Build history of the part. All positions in model axes, mm. Face numbers are marked on the shaded views. A direction names the side the tool comes from. Coordinates: 2 decimals unless noted, no trailing zeros. Loops run counter-clockwise (first coordinate to the right, second up) from the corner with the lowest first, then second, coordinate; pieces in that order, holes last.
Item 1: Drill centre lines: line 1 along Y through (x, z) = (-10.5, 21.5) (3 decimals); line 2 along Y through (x, z) = (35, 21) (3 decimals); line 3 along Y through (x, z) = (-15, 34.5) (3 decimals). Where is each one in solid material? Low to high.
Item 2: Cut at B-B (x = -7.5). List the corners of the cut face in (y, z) (3 decimals), and give its area (3 significant figures).
Item 3: 3-axis set-ups, long thin cutter, end or side, ignore diameter. For the marked faces 1 and 2: which of +Z, -Z, +X, -X, +Y, -Y reach the whole face in a straight line?
Item 4: Flat gauge pins, fed straight in: pin 1 (0.6 mm diameter, centred on x = 35.5, y = 30.5, fed in from +Z); pin 2 (4 mm diameter, centred on x = 41.275, y = -41.275, fed in from +Z). Where does each tip first touch, or does it go through?
Item 5: Cut at A-A (z = 8). Count the separate pieces of the cut face and the enclosed holes in it, and give its area (3 significant figures).
Item 6: Cut at C-C (y = 9). List the corners of the cut face in (x, z) (3 decimals), and give its area (3 significant figures).
Item 7: Mould opens along Y. For the marked faces 3, 4, 5 and 6 say: released by +Y, released by -Y, zero draft, split by the parting line, or undercut.
Item 8: Cut at D-D (z = 33). List the corners of the cut face in (x, y) (1 decimal).
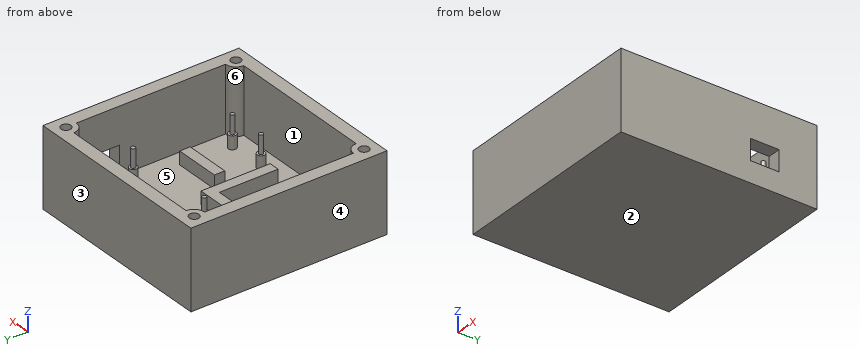
from build123d import *

# Parameters (mm, degrees)
SKETCH1_W           = 95.25
SKETCH1_H           = 95.25
BOSS_EXTRUDE1_DEPTH = 38.1
SHELL1_T            = -6.35
BOSS_EXTRUDE2_DEPTH = 31.75
SKETCH3_R           = 1.905
SKETCH3_R_2         = 1.016
BOSS_EXTRUDE3_DEPTH = 6.35
SKETCH4_R           = 1.016
BOSS_EXTRUDE4_DEPTH = 8.89
SKETCH5_R           = 1.905
SKETCH5_W           = 22.2885
SKETCH5_H           = 5.08
BOSS_EXTRUDE5_DEPTH = 6.35
SKETCH7_R           = 1.016
BOSS_EXTRUDE6_DEPTH = 8.89
SKETCH8_R           = 2.38125
CUT_EXTRUDE1_DEPTH  = 8.89
BOSS_EXTRUDE7_DEPTH = 6.35
SKETCH12_W          = 10.16
SKETCH12_H          = 13.97
CUT_EXTRUDE2_DEPTH  = 6.35


with BuildPart() as part:
    # Sketch1 → Boss-Extrude1 (new body)
    with BuildSketch(Plane.XY):
        Rectangle(SKETCH1_W, SKETCH1_H)
    extrude(amount=BOSS_EXTRUDE1_DEPTH)

    # Shell1
    shell1_openings = [part.faces().sort_by_distance(p)[0] for p in [
        (0, 0, 38.1),
    ]]
    offset(amount=SHELL1_T, openings=shell1_openings, kind=Kind.INTERSECTION)

    # Sketch2 → Boss-Extrude2 (add)
    with BuildSketch(Plane.XY.offset(38.1)):
        with BuildLine():
            Line((-41.275, 41.275), (-36.195, 41.275))
            ThreePointArc((-36.195, 41.275), (-37.682897552, 37.682897552), (-41.275, 36.195))
            Line((-41.275, 36.195), (-41.275, 41.275))
        make_face()
        with BuildLine():
            Line((36.195, 41.275), (41.275, 41.275))
            Line((41.275, 41.275), (41.275, 36.195))
            ThreePointArc((41.275, 36.195), (37.682897552, 37.682897552), (36.195, 41.275))
        make_face()
        with BuildLine():
            Line((41.275, -36.195), (41.275, -41.275))
            Line((41.275, -41.275), (36.195, -41.275))
            ThreePointArc((36.195, -41.275), (37.682897552, -37.682897552), (41.275, -36.195))
        make_face()
        with BuildLine():
            Line((-41.275, -36.195), (-41.275, -41.275))
            Line((-41.275, -41.275), (-36.195, -41.275))
            ThreePointArc((-36.195, -41.275), (-37.682897552, -37.682897552), (-41.275, -36.195))
        make_face()
    extrude(amount=-BOSS_EXTRUDE2_DEPTH)

    # Sketch3 → Boss-Extrude3 (add)
    with BuildSketch(Plane.XY.offset(6.35)):
        with Locations((35.015710728, 31.115)):
            Circle(SKETCH3_R)
        with Locations((-10.704289272, 31.115)):
            Circle(SKETCH3_R_2)
        with Locations((-10.704289272, 13.335)):
            Circle(SKETCH3_R)
        with Locations((35.015710728, 13.335)):
            Circle(SKETCH3_R)
    extrude(amount=BOSS_EXTRUDE3_DEPTH)

    # Sketch4 → Boss-Extrude4 (add)
    with BuildSketch(Plane.XY.offset(12.7)):
        with Locations((-10.704289272, 31.115)):
            Circle(SKETCH4_R)
        with Locations((-10.704289272, 13.335)):
            Circle(SKETCH4_R)
        with Locations((35.015710728, 31.115)):
            Circle(SKETCH4_R)
        with Locations((35.015710728, 13.335)):
            Circle(SKETCH4_R)
    extrude(amount=BOSS_EXTRUDE4_DEPTH)

    # Sketch5 → Boss-Extrude5 (add)
    with BuildSketch(Plane.XY.offset(6.35)):
        with Locations((13.2715, -32.385)):
            Circle(SKETCH5_R)
        with Locations((31.75, -32.385)):
            Circle(SKETCH5_R)
        with Locations((22.51075, -10.795)):
            Rectangle(SKETCH5_W, SKETCH5_H)
    extrude(amount=BOSS_EXTRUDE5_DEPTH)

    # Sketch7 → Boss-Extrude6 (add)
    with BuildSketch(Plane.XY.offset(12.7)):
        with Locations((13.2715, -32.385)):
            Circle(SKETCH7_R)
        with Locations((31.75, -32.385)):
            Circle(SKETCH7_R)
    extrude(amount=BOSS_EXTRUDE6_DEPTH)

    # Sketch8 → Cut-Extrude1 (cut)
    with BuildSketch(Plane.XY.offset(38.1)):
        with Locations((-41.275, 41.275)):
            Circle(SKETCH8_R)
        with Locations((41.275, 41.275)):
            Circle(SKETCH8_R)
        with Locations((41.275, -41.275)):
            Circle(SKETCH8_R)
        with Locations((-41.275, -41.275)):
            Circle(SKETCH8_R)
    extrude(amount=-CUT_EXTRUDE1_DEPTH, mode=Mode.SUBTRACT)

    # Sketch10 → Boss-Extrude7 (add)
    with BuildSketch(Plane.XY.offset(6.35)):
        Polygon((-30.8991, -30.607), (-30.8991, 2.9972), (5.0165, 2.9972), (5.0165, -30.607), (-0.0635, -30.607), (-0.0635, -2.0828), (-25.8191, -2.0828), (-25.8191, -30.607), align=None)
    extrude(amount=BOSS_EXTRUDE7_DEPTH)

    # Sketch12 → Cut-Extrude2 (cut)
    with BuildSketch(Plane(origin=(47.625, 0, 0), x_dir=(0, 0, -1), z_dir=(1, 0, 0))):
        with Locations((-15.24, 22.225)):
            Rectangle(SKETCH12_W, SKETCH12_H)
    extrude(amount=-CUT_EXTRUDE2_DEPTH, mode=Mode.SUBTRACT)


solid = part.part
Filled sheet:
1. line 1: y = -47.625 to -41.275, 12.34 to 14.33, 30.12 to 32.11, 41.275 to 47.625
1. line 2: y = -47.625 to -41.275, 12.319 to 14.351, 30.099 to 32.131, 41.275 to 47.625
1. line 3: y = -47.625 to -41.275, 41.275 to 47.625
2. outline: (-47.625, 0) - (47.625, 0) - (47.625, 38.1) - (41.275, 38.1) - (41.275, 6.35) - (2.997, 6.35) - (2.997, 12.7) - (-2.083, 12.7) - (-2.083, 6.35) - (-41.275, 6.35) - (-41.275, 38.1) - (-47.625, 38.1) - close
2. area: 1,040 mm2
3. face 1: +Z
3. face 2: -Z, +X, -X, +Y, -Y
4. pin 1: stops at z = 21.59
4. pin 2: stops at z = 29.21
5. separate pieces: 9
5. enclosed holes: 1
5. area: 2,980 mm2
6. outline: (-47.625, 0) - (47.625, 0) - (47.625, 38.1) - (41.275, 38.1) - (41.275, 6.35) - (-41.275, 6.35) - (-41.275, 38.1) - (-47.625, 38.1) - close
6. area: 1,010 mm2
7. face 3: released by +Y
7. face 4: zero draft
7. face 5: undercut
7. face 6: undercut
8. outline: (-47.6, -47.6) - (47.6, -47.6) - (47.6, 47.6) - (-47.6, 47.6) - close; hole circle Ø4.8 at (-41.3, -41.3); hole circle Ø4.8 at (-41.3, 41.3); hole (-41.3, -36.2) arc R5.1 cw to (-36.2, -41.3) - (36.2, -41.3) arc R5.1 cw to (41.3, -36.2) - (41.3, 36.2) arc R5.1 cw to (36.2, 41.3) - (-36.2, 41.3) arc R5.1 cw to (-41.3, 36.2) - close; hole circle Ø4.8 at (41.3, -41.3); hole circle Ø4.8 at (41.3, 41.3)
